from build123d import *

# Parameters (mm, degrees)
SKETCH1_R           = 15.9
SKETCH1_R_2         = 1.65
SKETCH1_R_3         = 2.925
SKETCH1_R_4         = 1.5
BOSS_EXTRUDE1_DEPTH = 3.7
SKETCH2_R           = 7.347175161
SKETCH2_R_2         = 7.491995358
CUT_EXTRUDE1_DEPTH  = 2.1


with BuildPart() as part:
    # Sketch1 → Boss-Extrude1 (new body)
    with BuildSketch(Plane.XY):
        with Locations((169.819947444, 173.617651357)):
            Circle(SKETCH1_R)
        with Locations((181.069947444, 173.617651357)):
            Circle(SKETCH1_R_2, mode=Mode.SUBTRACT)
        with Locations((158.569947444, 173.617651357)):
            Circle(SKETCH1_R_3, mode=Mode.SUBTRACT)
        with Locations((164.194947444, 163.874865564)):
            Circle(SKETCH1_R_2, mode=Mode.SUBTRACT)
        with Locations((164.194947444, 183.360437149)):
            Circle(SKETCH1_R_2, mode=Mode.SUBTRACT)
        with Locations((175.444947444, 183.360437149)):
            Circle(SKETCH1_R_3, mode=Mode.SUBTRACT)
        with Locations((175.444947444, 163.874865564)):
            Circle(SKETCH1_R_3, mode=Mode.SUBTRACT)
        with Locations((169.819947444, 173.617651357)):
            Circle(SKETCH1_R_4, mode=Mode.SUBTRACT)
    extrude(amount=BOSS_EXTRUDE1_DEPTH)

    # Sketch2 → Cut-Extrude1 (cut)
    with BuildSketch(Plane(origin=(0, 0, 0), x_dir=(-1, 0, 0), z_dir=(0, 0, -1))):
        with Locations((-169.819947444, 173.617651357)):
            Circle(SKETCH2_R)
        with Locations((-158.569947444, 173.617651357)):
            Circle(SKETCH2_R_2)
        with Locations((-175.444947444, 163.874865564)):
            Circle(SKETCH2_R_2)
        with Locations((-175.444947444, 183.360437149)):
            Circle(SKETCH2_R_2)
    extrude(amount=-CUT_EXTRUDE1_DEPTH, mode=Mode.SUBTRACT)


solid = part.part
Source: CAD feature listing. Evaluate the final solid. Frame: model axes, mm. A direction names the side the tool comes from. Round coordinates to 2 decimals unless told otherwise and drop trailing zeros. Loops run counter-clockwise (first coordinate to the right, second up) from the corner with the lowest first, then second, coordinate; pieces in that order, holes last. Notation, with made-up numbers: M 39,29 L 43,29 A23 ccw 43,58 Z; hole C 32,-37 d2. An arc over 180 degrees is marked long. Return JSON: item names as keys, results as strings. Group by question number.
1. Pin query (flat end, axial travel): pin 1 (9.5 mm diameter, centred on x = 158.57, y = 173.62, fed in from -Z); pin 2 (1.5 mm diameter, centred on x = 173, z = 2.5, fed in from -Y); pin 3 (3 mm diameter, centred on x = 181.07, y = 173.62, fed in from +Z). Return the tip coordinate at first contact, or that it passes through.
2. Section query D-D on z = 3.3. Output: boundary loops of the cut face in (x, y) (3 decimals).
3. Reachability of faces 5 (the face through (168.316, 161.57, 1.035)), 6 (the face through (181.006, 178.34, 1.035)), 7 (the face through (177.167, 173.651, 1.035)) from +Z, -Z, +X, -X, +Y, -Y: full face, straight path, thin tool, end or side. Return the list, or none.
4. Mould query, pull axis X, two halves, no side actions, for faces 1 (the face through (168.276, 185.536, 1.035)), 2 (the face through (179.42, 173.69, 1.82)), 3 (the face through (163, 162, 0)), 4 (the face through (184.51, 167.53, 1.82)). Classes: released by +X, released by -X, zero draft, split by the parting line, or undercut.
5. Section query C-C on y = 184. Output: boundary loops of the cut face in (x, z), and give its area (3 significant figures).
6. Material intervals for line 1 along X through (y, z) = (172.5, 2.4); line 2 along Y through (x, z) = (163, 0.2); line 3 along Y through (x, z) = (165.5, 2), sorted ascending. Write a range as from..to.
7. Section query B-B on x = 163. Output: boundary loops of the cut face in (y, z), and give its area (3 significant figures).
8. Section query A-A on z = 0.4. Output: boundary loops of the cut face in (x, y), and give its area (3 significant figures).
Checks:
{
 "1": {"pin 1": "stops at z = 2.1", "pin 2": "stops at y = 157.9", "pin 3": "passes through"},
 "2": {"outline": "C 169.82,173.618 d31.8; hole C 158.57,173.618 d5.85; hole C 164.195,163.875 d3.3; hole C 164.195,183.36 d3.3; hole C 169.82,173.618 d3; hole C 175.445,163.875 d5.85; hole C 175.445,183.36 d5.85; hole C 181.07,173.618 d3.3"},
 "3": {"face 5": "-Z", "face 6": "-Z, +Y", "face 7": "-Z, -X"},
 "4": {"face 1": "undercut", "face 2": "undercut", "face 3": "zero draft", "face 4": "split by the parting line"},
 "5": {"outline": "M 157.78,0 L 162.67,0 L 162.67,3.7 L 157.78,3.7 Z; M 165.72,0 L 167.98,0 L 167.98,2.1 L 172.59,2.1 L 172.59,3.7 L 165.72,3.7 Z; M 178.3,2.1 L 181.86,2.1 L 181.86,3.7 L 178.3,3.7 Z", "area": "39.6 mm²"},
 "6": {"line 1": "x = 153.96..155.87, 161.27..168.82, 170.82..179.86, 182.28..185.68", "line 2": "y = 159.25..162.74, 165.01..167.58, 179.66..182.22, 184.5..187.98", "line 3": "y = 158.32..162.87, 164.88..167.67, 179.56..182.35, 184.37..188.92"},
 "7": {"outline": "M 159.25,0 L 162.74,0 L 162.74,3.7 L 159.25,3.7 Z; M 165.01,0 L 167.58,0 L 167.58,2.1 L 179.66,2.1 L 179.66,0 L 182.22,0 L 182.22,3.7 L 165.01,3.7 Z; M 184.5,0 L 187.98,0 L 187.98,3.7 L 184.5,3.7 Z", "area": "64.1 mm²"},
 "8": {"outline": "M 155.45,166.8 A15.9 ccw 171.1,157.77 A7.49 cw 168.39,166.41 A7.35 cw 164.29,168.78 A7.49 cw Z; M 155.45,180.43 A7.49 cw 164.29,178.46 A7.35 cw 168.39,180.83 A7.49 cw 171.1,189.47 A15.9 ccw Z; M 176.77,171.25 A7.49 cw 182.9,164.58 A15.9 ccw 182.9,182.65 A7.49 cw 176.77,175.99 A7.35 cw Z; hole C 164.19,163.87 d3.3; hole C 164.19,183.36 d3.3; hole C 181.07,173.62 d3.3", "area": "228 mm²"}
}
